Work out the finished part from the listing and answer in its coordinate system (mm). Face numbers are marked on the shaded views. Give positions to 0.01 mm unless a question says otherwise; leave off trailing zeros. Write each loop counter-clockwise with the first axis right and the second up, starting at its lowest first coordinate (ties: lowest second). Pieces come first, ordered by that corner, then holes. Notation, with made-up numbers: (60.25, 1) - (95.25, 1) arc R17 ccw to (95.25, 9) - close; hole circle Ø2 at (-15, 63.5). An arc over 180 degrees is marked (long way). Write item = value, one per line.
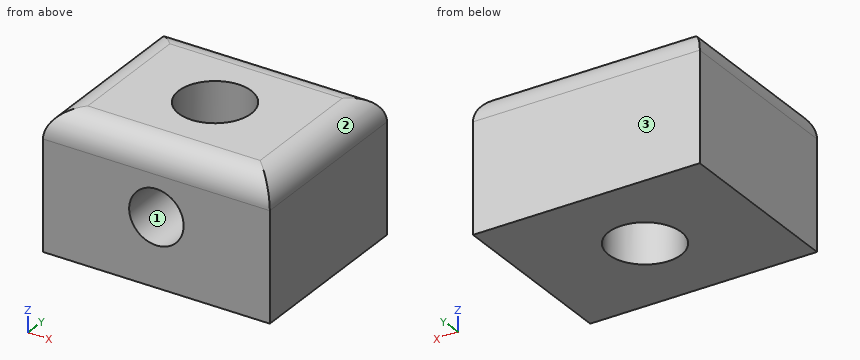
from build123d import *

# Parameters (mm, degrees)
F0_W     = 25
F0_H     = 20
F0_R     = 4
F1_DEPTH = 15
F2_R     = 3
F3_DEPTH = 10
F4_R     = 3


with BuildPart() as f1:
    # F0 (on Top) → F1 (new body)
    with BuildSketch(Plane.XY):
        with Locations((12.5, -10)):
            Rectangle(F0_W, F0_H)
        with Locations((12.5, -10)):
            Circle(F0_R, mode=Mode.SUBTRACT)
    extrude(amount=F1_DEPTH)

    # F2 (on face) → F3 (cut)
    with BuildSketch(Plane.XZ.offset(20)):
        with Locations((12.5, 7.5)):
            Circle(F2_R)
    extrude(amount=-F3_DEPTH, mode=Mode.SUBTRACT)

    # F4
    f4_edges = [f1.edges().sort_by_distance(p)[0] for p in [
        (0, -10, 15),
        (12.5, 0, 15),
        (25, -10, 15),
        (12.5, -20, 15),
    ]]
    fillet(f4_edges, radius=F4_R)


solid = f1.part
1. Straight lines are drawn through the part: line 1 (Y direction, x = 12.5, z = 4.25); line 2 (X direction, y = -15, z = 7.5); line 3 (Y direction, x = 12.5, z = 9). For each, find the intervals that lie inside material, in ascending order.
Solution:
line_1 = -20 to -14, -6 to 0
line_2 = 0 to 9.5, 15.5 to 25
line_3 = -6 to 0
2. For a pull along X with two mould halves and no side action, classify the marked faces 1, 2 and 3 as pulls with the +X half, pulls with the -X half, needs draft (parallel to the pull), parting line crosses it, or undercut.
Solution:
face_1 = undercut
face_2 = pulls with the +X half
face_3 = needs draft
3. Find section C-C, the plane y = -18.25. Give the vertices of the cut face in (x, z), then the cut area to 3 significant figures.
Solution:
outline = (0, 0) - (25, 0) - (25, 12) arc R3 ccw to (23.25, 14.73) - (1.75, 14.73) arc R3 ccw to (0, 12) - close; hole circle Ø6 at (12.5, 7.5)
area = 337 mm^2
4. Find section A-A, the plane x = 12.5. Give the vertices of the cut face in (y, z).
Solution:
outline = (-20, 0) - (-14, 0) - (-14, 4.5) - (-20, 4.5) - close; (-20, 10.5) - (-14, 10.5) - (-14, 15) - (-17, 15) arc R3 ccw to (-20, 12) - close; (-6, 0) - (0, 0) - (0, 12) arc R3 ccw to (-3, 15) - (-6, 15) - close
5. Find section D-D, the plane z = 7.5. Give the vertices of the cut face in (x, y), then the cut area to 3 significant figures.
Solution:
outline = (0, -20) - (9.5, -20) - (9.5, -12.65) arc R4 cw (long way) to (15.5, -12.65) - (15.5, -20) - (25, -20) - (25, 0) - (0, 0) - close
area = 411 mm^2
6. Find section B-B, the plane y = -10. Give the vertices of the cut face in (x, z), then the cut area to 3 significant figures.
Solution:
outline = (0, 0) - (8.5, 0) - (8.5, 15) - (3, 15) arc R3 ccw to (0, 12) - close; (16.5, 0) - (25, 0) - (25, 12) arc R3 ccw to (22, 15) - (16.5, 15) - close
area = 251 mm^2
